Source: CAD feature listing. Evaluate the final solid. Frame: model axes, mm. A direction names the side the tool comes from. Give positions to 0.01 mm unless a question says otherwise; leave off trailing zeros. Loops run counter-clockwise (first coordinate to the right, second up) from the corner with the lowest first, then second, coordinate; pieces in that order, holes last. Notation, with made-up numbers: M -23.5,66 L 31.5,66 A23 ccw 31.5,103 Z; hole C -21.75,34 d3. An arc over 180 degrees is marked long. Answer in a Markdown table with one row per item.
```python
from build123d import *

# Parameters (mm, degrees)
SKETCH1_R           = 55.5
SKETCH1_R_2         = 40
BOSS_EXTRUDE1_DEPTH = 2
BOSS_EXTRUDE2_DEPTH = 2
CIRPATTERN1_COUNT   = 30


with BuildPart() as part:
    # Sketch1 → Boss-Extrude1 (new body)
    with BuildSketch(Plane.YZ):
        with Locations(Location((0, 0, 0), (0, 0, 270))):
            Circle(SKETCH1_R)
        with Locations(Location((0, 0, 0), (0, 0, 270))):
            Circle(SKETCH1_R_2, mode=Mode.SUBTRACT)
    extrude(amount=BOSS_EXTRUDE1_DEPTH)

    # Sketch1_3 → Boss-Extrude2 (add)
    with BuildSketch(Plane.YZ):
        with BuildLine():
            Line((-2, 39.949968711), (-2, 38))
            Line((-2, 38), (2, 38))
            Line((2, 38), (2, 39.949968711))
            ThreePointArc((2, 39.949968711), (0, 40), (-2, 39.949968711))
        make_face()
    boss_extrude2 = extrude(amount=BOSS_EXTRUDE2_DEPTH)

    # CirPattern1: Boss-Extrude2 ×30 about axis
    cirpattern1_axis = Axis((0, 0, 0), (1, 0, 0))
    for i in range(1, CIRPATTERN1_COUNT):
        add(boss_extrude2.rotate(cirpattern1_axis, i * 360 / CIRPATTERN1_COUNT))


solid = part.part
```
1) Pin query (flat end, axial travel): pin 1 Ø1 at (x, z) = (1.5, -39) entering from -Y (3 decimals); pin 2 Ø1 at (x, z) = (1, 39.5) entering from -Y; pin 3 Ø1 at (x, y) = (0.5, 40.5) entering from -Z. Return the tip coordinate at first contact, or that it passes through.
Reply:
| item | result |
|---|---|
| pin 1 | stops at y = -39.975 |
| pin 2 | stops at y = -39.49 |
| pin 3 | stops at z = -38.47 |
2) Section B-B, the plane y = 0. Return loops of the section in (x, z), then the cut area to 3 significant figures.
Reply:
| item | result |
|---|---|
| outline | M 0,-55.5 L 2,-55.5 L 2,-38 L 0,-38 Z; M 0,38 L 2,38 L 2,55.5 L 0,55.5 Z |
| area | 70.0 mm² |
3) Section C-C, the plane y = 47. Return loops of the section in (x, z).
Reply:
| item | result |
|---|---|
| outline | M 0,-29.52 L 2,-29.52 L 2,29.52 L 0,29.52 Z |
4) Pull-direction query (Y, two-part tool) for faces 3 (the cylindrical face through (0.99, -26.74, 29.75)), 4 (the flat face through (2, -36, 13)), 5 (the cylindrical face through (0.986, 46.798, -29.836)); classes: released by +Y, released by -Y, zero draft, split by the parting line, or undercut.
Reply:
| item | result |
|---|---|
| face 3 | undercut |
| face 4 | zero draft |
| face 5 | split by the parting line |
5) Set-up query: faces 1 (the flat face through (0.986, 28.258, -25.406)), 2 (the flat face through (0, -36, 13)). Return all of +Z, -Z, +X, -X, +Y, -Y with unobstructed straight access to the full face (end or side cutting, diameter ignored); none if empty.
Reply:
| item | result |
|---|---|
| face 1 | +X, -X |
| face 2 | +Z, -Z, -X, +Y, -Y |
6) Material intervals for L1, parallel to Y at x = 1.1, z = 24.5; L2, parallel to Y at x = 1.65, z = 39; L3, parallel to Z at x = 1.55, y = -38.5 (1 decimal), sorted ascending.
Reply:
| item | result |
|---|---|
| L1 | y = -49.8 to -31.62, -30.2 to -29.07, 29.07 to 30.2, 31.62 to 49.8 |
| L2 | y = -39.49 to -6.25, -2 to 2, 6.25 to 39.49 |
| L3 | z = -40 to -10.4, -6.1 to -2, 2 to 6.1, 10.4 to 40 |
7) Section A-A, the plane z = 0. Return loops of the section in (x, y).
Reply:
| item | result |
|---|---|
| outline | M 0,-55.5 L 2,-55.5 L 2,-40 L 0,-40 Z; M 0,40 L 2,40 L 2,55.5 L 0,55.5 Z |
